Design review of the part built by this model. Coordinates are the model's own, in mm. A direction names the side the tool comes from. Round coordinates to 2 decimals unless told otherwise and drop trailing zeros. Order: outer loops, then holes, each group sorted by start corner. A loop starts at its lowest first (then second) coordinate and runs counter-clockwise, first axis right, second up. Notation, with made-up numbers: M 34.5,2 L 43.5,2 A33 ccw 43.5,30 Z; hole C -40,60.25 d4. An arc over 180 degrees is marked long. Use a Markdown table: item, result. Add a question column.
(1) Machinability: for faces 5 (the face through (-10, 0, 6)), 6 (the face through (20.14, 20.1, 2.96)), which of the approach directions +Z, -Z, +X, -X, +Y, -Y give a long, thin tool a straight path to every point of the face, cutting with its end or side? Answer none if there is none.
(2) Take a section at A-A (y = 16.5). Write out the cut boundary in (x, z).
(3) For pin 1 (3 mm diameter, centred on x = -16.5, y = 16.5, fed in from +Z); pin 2 (1.5 mm diameter, centred on x = -13, y = -9.5, fed in from +Z); pin 3 (8 mm diameter, centred on x = 12.5, y = 14, fed in from -Z); pin 4 (6 mm diameter, centred on x = 6, z = 3.5, fed in from -Y), all flat-tipped, find the tip position at first contact; note any pin that passes through.
(4) To check wall thickness, follow probe 1 along Y at (x, z) = (-16.5, 2.5); probe 2 along Z at (x, y) = (-17, -10); probe 3 along Y at (x, z) = (2, 13.5). State the ranges of each line that lie inside material, in increasing order. Write a range as from..to.
(5) The part is to be moulded in two halves that separate along X. For faces 1 (the face through (0, -3, 16)), 2 (the face through (-0.596, -2.685, 7.888)), 3 (the face through (-16.728, -14.765, 2.958)), 4 (the face through (-1.009, 7.684, 10.93)), say which applies: released by +X, released by -X, zero draft, split by the parting line, or undercut.
(6) Take a section at C-C (x = 16.5). Write out the cut boundary in (y, z), then the cut area to 3 significant figures.
(7) Take a section at D-D (y = -16.5). Write out the cut boundary in (x, z), then the cut area to 3 significant figures.
```python
from build123d import *

# Parameters (mm, degrees)
F0_R     = 1.75
F0_R_2   = 2.75
F1_DEPTH = 6
F3_DEPTH = 25
F4_R     = 7.75
F4_R_2   = 2.75
F5_DEPTH = 10


with BuildPart() as f1:
    # F0 (on Top) → F1 (new body)
    with BuildSketch(Plane.XY):
        with BuildLine():
            ThreePointArc((21, 18), (20.12132, 20.12132), (18, 21))
            Line((18, 21), (-18, 21))
            ThreePointArc((-18, 21), (-20.12132, 20.12132), (-21, 18))
            Line((-21, 18), (-21, -18))
            ThreePointArc((-21, -18), (-20.12132, -20.12132), (-18, -21))
            Line((-18, -21), (18, -21))
            ThreePointArc((18, -21), (20.12132, -20.12132), (21, -18))
            Line((21, -18), (21, 18))
        make_face()
        with Locations((-16.5, -16.5)):
            Circle(F0_R, mode=Mode.SUBTRACT)
        with Locations((16.5, -16.5)):
            Circle(F0_R, mode=Mode.SUBTRACT)
        with Locations((-16.5, 16.5)):
            Circle(F0_R, mode=Mode.SUBTRACT)
        Circle(F0_R_2, mode=Mode.SUBTRACT)
        with Locations((16.5, 16.5)):
            Circle(F0_R, mode=Mode.SUBTRACT)
    extrude(amount=F1_DEPTH)

    # F2 (on face) → F3 (cut)
    with BuildSketch(Plane.XY.offset(6)):
        Polygon((21, 0), (0, -21), (21, -21), align=None)
    extrude(amount=-F3_DEPTH, mode=Mode.SUBTRACT)

    # F4 (on face) → F5 (join)
    with BuildSketch(Plane.XY.offset(6)):
        Circle(F4_R)
        Circle(F4_R_2, mode=Mode.SUBTRACT)
    extrude(amount=F5_DEPTH)


solid = f1.part
```
Verdict:
| question | item | result |
|---|---|---|
| 1 | face 5 | +Z |
| 1 | face 6 | +Z, -Z, +X, +Y |
| 2 | outline | M -21,0 L -18.25,0 L -18.25,6 L -21,6 Z; M -14.75,0 L 14.75,0 L 14.75,6 L -14.75,6 Z; M 18.25,0 L 21,0 L 21,6 L 18.25,6 Z |
| 3 | pin 1 | passes through |
| 3 | pin 2 | stops at z = 6 |
| 3 | pin 3 | stops at z = 0 |
| 3 | pin 4 | stops at y = -18 |
| 4 | probe 1 | y = -21..-18.25, -14.75..14.75, 18.25..21 |
| 4 | probe 2 | z = 0..6 |
| 4 | probe 3 | y = -7.49..-1.89, 1.89..7.49 |
| 5 | face 1 | zero draft |
| 5 | face 2 | undercut |
| 5 | face 3 | undercut |
| 5 | face 4 | split by the parting line |
| 6 | outline | M -4.5,0 L 14.75,0 L 14.75,6 L -4.5,6 Z; M 18.25,0 L 21,0 L 21,6 L 18.25,6 Z |
| 6 | area | 132 mm^2 |
| 7 | outline | M -21,0 L -18.25,0 L -18.25,6 L -21,6 Z; M -14.75,0 L 4.5,0 L 4.5,6 L -14.75,6 Z |
| 7 | area | 132 mm^2 |
